```python
from build123d import *

# Parameters (mm, degrees)
BOSS_EXTRUDE1_DEPTH        = 12
SKETCH2_R                  = 10
BOSS_EXTRUDE2_DEPTH        = 13
F_12_0MM_DOWEL_HOLE1_D     = 12
F_12_0MM_DOWEL_HOLE1_DEPTH = 15
F_12_0MM_DOWEL_HOLE1_TIP   = 3.605163714
F_4_0MM_DOWEL_HOLE1_D      = 4
M2X0_4_TAPPED_HOLE1_REACH  = 41.205
M2X0_4_TAPPED_HOLE1_BORE_R = 0.8
SKETCH11_R                 = 3
CUT_EXTRUDE1_DEPTH         = 1
CIRPATTERN1_COUNT          = 2
CUT_EXTRUDE2_START         = -3
SKETCH13_R                 = 10.893382682
SKETCH13_R_2               = 9
CUT_EXTRUDE2_DEPTH         = 3


# Read off the part's stored shape, not the designer's step: M18x1.5 Machine Threads Stud1
with BuildPart() as part:
    # Sketch1 → Boss-Extrude1 (new body)
    with BuildSketch(Plane.XY):
        Polygon((6.92820323, 12), (-6.92820323, 12), (-13.856406461, 0), (-6.92820323, -12), (6.92820323, -12), (13.856406461, 0), align=None)
    extrude(amount=BOSS_EXTRUDE1_DEPTH)

    # Sketch2 → Boss-Extrude2 (add)
    with BuildSketch(Plane.XY.offset(12)):
        with Locations(Location((0, 0, 0), (0, 0, 180))):
            Circle(SKETCH2_R)
    extrude(amount=BOSS_EXTRUDE2_DEPTH)

    # Ø12.0mm Dowel Hole1
    with Locations(Plane(origin=(0, 0, 0), x_dir=(-1, 0, 0), z_dir=(0, 0, -1))):
        with Locations((0, 0)):
            Hole(F_12_0MM_DOWEL_HOLE1_D / 2, depth=F_12_0MM_DOWEL_HOLE1_DEPTH)
            with Locations((0, 0, -(F_12_0MM_DOWEL_HOLE1_DEPTH + F_12_0MM_DOWEL_HOLE1_TIP / 2))):  # 118° drill point
                Cone(0, F_12_0MM_DOWEL_HOLE1_D / 2, F_12_0MM_DOWEL_HOLE1_TIP, mode=Mode.SUBTRACT)

    # Ø4.0mm Dowel Hole1 (through all)
    with Locations(Plane(origin=(0, 12, 0), x_dir=(1, 0, 0), z_dir=(0, 1, 0))):
        with Locations((0, -8)):
            Hole(F_4_0MM_DOWEL_HOLE1_D / 2)

    # M2x0.4 Tapped Hole1 bore → M2x0.4 Tapped Hole1 (cut, up to next)
    with BuildSketch(Plane(origin=(10.392304845, 6, 0), x_dir=(0, 0, -1), z_dir=(0.8660254037844387, 0.49999999999999994, 0)), mode=Mode.PRIVATE) as m2x0_4_tapped_hole1_sk1:
        with Locations((-2, 0)):
            Circle(M2X0_4_TAPPED_HOLE1_BORE_R)
    m2x0_4_tapped_hole1_tool1 = extrude(m2x0_4_tapped_hole1_sk1.sketch, amount=-M2X0_4_TAPPED_HOLE1_REACH, mode=Mode.PRIVATE) & part.part
    add(m2x0_4_tapped_hole1_tool1.solids().sort_by_distance((10.392305, 6, 2))[0], mode=Mode.SUBTRACT)

    # Sketch11 → Cut-Extrude1 (cut)
    with BuildSketch(Plane.XZ.offset(12)):
        with Locations((0, 8)):
            Circle(SKETCH11_R)
    cut_extrude1 = extrude(amount=-CUT_EXTRUDE1_DEPTH, mode=Mode.SUBTRACT)

    # CirPattern1: Cut-Extrude1 ×2 about axis
    cirpattern1_axis = Axis((0, 0, 25), (0, 0, -1))
    for i in range(1, CIRPATTERN1_COUNT):
        add(cut_extrude1.rotate(cirpattern1_axis, i * 360 / CIRPATTERN1_COUNT), mode=Mode.SUBTRACT)

    # M18x1.5 Machine Threads Stud1 outline → M18x1.5 Machine Threads Stud1 (revolve, cut)
    with BuildSketch(Plane.XZ):
        Polygon((10, 25), (8.172, 25), (9, 24.172), (9, 15), (10, 15), align=None)
    revolve(axis=Axis((0, 0, 0), (0, 0, 1)), mode=Mode.SUBTRACT)

    # Sketch13 → Cut-Extrude2 (cut)
    with BuildSketch(Plane.XY.offset(15).offset(CUT_EXTRUDE2_START)):
        Circle(SKETCH13_R)
        with Locations(Location((0, 0, 0), (0, 0, 180))):
            Circle(SKETCH13_R_2, mode=Mode.SUBTRACT)
    extrude(amount=CUT_EXTRUDE2_DEPTH, mode=Mode.SUBTRACT)


solid = part.part
```
Input: part model. Units: mm. Frame: model coordinates. A direction names the side the tool comes from. Give positions to 0.01 mm unless a question says otherwise; leave off trailing zeros. Loops run counter-clockwise (first coordinate to the right, second up) from the corner with the lowest first, then second, coordinate; pieces in that order, holes last. Notation, with made-up numbers: M 0,41 L 24,41 A5 ccw 24,49 Z; hole C 42.25,24 d11. An arc over 180 degrees is marked long. Answer as CSV lines item,"result". Start each with the question number.
1. Section C-C on z = 21.75. Return loops of the section in (x, y), plus the area to 3 significant figures.
2. Section D-D on x = -11.5. Return loops of the section in (y, z).
3. Section A-A on z = 8. Return loops of the section in (x, y), plus the area to 3 significant figures.
4. Reachability of faces 4 (the face through (-2, 11, 7)), 5 (the face through (5.54, -2.3, 7.6)), 6 (the face through (1.61, -11.51, 10.53)) from +Z, -Z, +X, -X, +Y, -Y: full face, straight path, thin tool, end or side. Return the list, or none.
5. Section B-B on y = 9.5. Return loops of the section in (x, z), plus the area to 3 significant figures.
6. Line query: L1, parallel to Z at x = 0, y = 11.65; L2, parallel to X at y = -8.4, z = 8; L3, parallel to Z at x = -6.75, y = 10.75. Output: solid intervals per line, ascending.
7. Pull-direction query (X, two-part tool) for faces 1 (the face through (9, 3, 12)), 2 (the face through (2, -11, 7)), 3 (the face through (-10.44, -5.92, 5.92)); classes: released by +X, released by -X, zero draft, split by the parting line, or undercut.
8. Pin query (flat end, axial travel): P1, Ø2, axis at y = -9, z = 9.5, coming from the +X side; P2, Ø8, axis at y = 4.5, z = 20.5, coming from the +X side; P3, Ø6, axis at y = 6.5, z = 17, coming from the -X side; P4, Ø2.5, axis at x = 0, z = 8, coming from the +Y side. Return the tip coordinate at first contact, or that it passes through.
Computed values:
1,outline,"C 0,0 d18"
1,area,"254 mm²"
2,outline,"M -4.08,0 L 4.08,0 L 4.08,12 L -4.08,12 Z"
3,outline,"M -13.86,0 L -6.93,-12 L -3,-12 L -3,-11 L -2,-11 L -2,-5.66 A6 cw -2,5.66 L -2,11 L -3,11 L -3,12 L -6.93,12 Z; M 2,-11 L 3,-11 L 3,-12 L 6.93,-12 L 13.86,0 L 6.93,12 L 3,12 L 3,11 L 2,11 L 2,5.66 A6 cw 2,-5.66 Z"
3,area,"333 mm²"
4,face 4,"+Y"
4,face 5,"-Z"
4,face 6,"-Y"
5,outline,"M -8.37,0 L 8.37,0 L 8.37,12 L -8.37,12 Z; hole C 0,8 d4"
5,area,"188 mm²"
6,L1,"z = 0 to 5, 11 to 12"
6,L2,"x = -9.01 to -2, 2 to 9.01"
6,L3,"z = 0 to 12"
7,face 1,"zero draft"
7,face 2,"undercut"
7,face 3,"released by -X"
8,P1,"stops at x = 9.24"
8,P2,"stops at x = 8.99"
8,P3,"stops at x = -8.29"
8,P4,"passes through"
